from build123d import *

# Parameters (mm, degrees)
SKETCH_1_R          = 12.5
SKETCH_1_R_2        = 3.05
EXTRUDE_1_DEPTH     = 8
SKETCH_2_R          = 1.6
CUT_EXTRUDE_4_DEPTH = 12.5
SKETCH_3_R          = 5.05
EXTRUDE_2_DEPTH     = 6
SKETCH_4_R          = 18
EXTRUDE_3_DEPTH     = 2
FILLET_2_R          = 30
FILLET_1_R          = 1
EXTRUDE_4_DEPTH     = 10
FILLET_3_R          = 4
SKETCH_6_R          = 3.05
CUT_EXTRUDE_5_DEPTH = 14
CUT_EXTRUDE_6_REACH = 81.906


with BuildPart() as part:
    # 草图1 → 凸台-拉伸1 (new body)
    with BuildSketch(Plane(origin=(0, 0, 0), x_dir=(1, 0, 0), z_dir=(0, 1, 0))):
        with Locations(Location((0, 0, 0), (0, 0, 270))):
            Circle(SKETCH_1_R)
        with Locations(Location((0, 0, 0), (0, 0, 270))):
            Circle(SKETCH_1_R_2, mode=Mode.SUBTRACT)
    extrude(amount=EXTRUDE_1_DEPTH)

    # 草图2 → 切除-拉伸4 (cut, symmetric)
    with BuildSketch(Plane.XY):
        with Locations((0, 3.3)):
            Circle(SKETCH_2_R)
    extrude(amount=CUT_EXTRUDE_4_DEPTH, both=True, mode=Mode.SUBTRACT)

    # 草图3 → 凸台-拉伸2 (add)
    with BuildSketch(Plane(origin=(0, 8, 0), x_dir=(1, 0, 0), z_dir=(0, 1, 0))):
        with BuildLine():
            Line((5.416666667, 24.406141076), (62.6, 11.714947716))
            ThreePointArc((62.6, 11.714947716), (71.918087828, 1.399708015), (65.243514508, -10.793773928))
            Line((65.243514508, -10.793773928), (36, -25))
            Line((36, -25), (0, -25))
            ThreePointArc((0, -25), (-24.851091796, 2.724561717), (5.416666667, 24.406141076))
        make_face()
        with Locations(Location((60, 0, 0), (0, 0, 270))):
            Circle(SKETCH_3_R, mode=Mode.SUBTRACT)
    extrude(amount=EXTRUDE_2_DEPTH)

    # 草图4 → 凸台-拉伸3 (add)
    with BuildSketch(Plane.XZ.offset(-8)):
        with Locations(Location((0, 0, 0), (0, 0, 90))):
            Circle(SKETCH_4_R)
    extrude(amount=EXTRUDE_3_DEPTH)

    # 圆角2
    fillet_2_edges = [part.edges().sort_by_distance(p)[0] for p in [
        (36, 11, 25),
    ]]
    fillet(fillet_2_edges, radius=FILLET_2_R)

    # 圆角1
    fillet_1_edges = [part.edges().sort_by_distance(p)[0] for p in [
        (0, 6, -18),
    ]]
    fillet(fillet_1_edges, radius=FILLET_1_R)

    # 草图5 → 凸台-拉伸4 (add)
    with BuildSketch(Plane(origin=(0, 14, 0), x_dir=(1, 0, 0), z_dir=(0, 1, 0))):
        with BuildLine():
            Line((0, 0), (-25, 0))
            ThreePointArc((-25, 0), (-23.096988313, -9.567085809), (-17.67766953, -17.67766953))
            Line((-17.67766953, -17.67766953), (0, 0))
        make_face()
    extrude(amount=EXTRUDE_4_DEPTH)

    # 圆角3
    fillet_3_edges = [part.edges().sort_by_distance(p)[0] for p in [
        (0, 19, 0),
    ]]
    fillet(fillet_3_edges, radius=FILLET_3_R)

    # 草图6 → 切除-拉伸5 (cut)
    with BuildSketch(Plane.XZ):
        with Locations(Location((0, 0, 0), (0, 0, 90))):
            Circle(SKETCH_6_R)
    extrude(amount=-CUT_EXTRUDE_5_DEPTH, mode=Mode.SUBTRACT)

    # 切除-拉伸6: up to this face of the body (flat: up to its plane)
    cut_extrude_6_end = Plane(part.part.faces().sort_by_distance((0, 6, -16.519167389))[0])
    # 草图8 → 切除-拉伸6 (cut, up to the picked face)
    with BuildSketch(Plane.XZ, mode=Mode.PRIVATE) as cut_extrude_6_sk1:
        with BuildLine():
            ThreePointArc((5.937171044, 11), (0, 12.5), (-5.937171044, 11))
            Line((-5.937171044, 11), (5.937171044, 11))
        make_face()
    cut_extrude_6_tool1 = split(extrude(cut_extrude_6_sk1.sketch, amount=-CUT_EXTRUDE_6_REACH, mode=Mode.PRIVATE), bisect_by=cut_extrude_6_end, keep=Keep.BOTH, mode=Mode.PRIVATE)
    # 草图8 → 切除-拉伸6 (cut, up to the picked face)
    with BuildSketch(Plane.XZ, mode=Mode.PRIVATE) as cut_extrude_6_sk2:
        with BuildLine():
            Line((5.937171044, -11), (-5.937171044, -11))
            ThreePointArc((-5.937171044, -11), (0, -12.5), (5.937171044, -11))
        make_face()
    cut_extrude_6_tool2 = split(extrude(cut_extrude_6_sk2.sketch, amount=-CUT_EXTRUDE_6_REACH, mode=Mode.PRIVATE), bisect_by=cut_extrude_6_end, keep=Keep.BOTH, mode=Mode.PRIVATE)
    add(cut_extrude_6_tool1.solids().sort_by(Axis((0, 0, 11.603197), (0, 1, 0)))[0], mode=Mode.SUBTRACT)
    add(cut_extrude_6_tool2.solids().sort_by(Axis((0, 0, -11.603197), (0, 1, 0)))[0], mode=Mode.SUBTRACT)


solid = part.part
The listing builds one solid part. Answer for the finished solid, in the listing's coordinates (mm). A direction names the side the tool comes from. Give positions to 0.01 mm unless a question says otherwise; leave off trailing zeros. Loops run counter-clockwise (first coordinate to the right, second up) from the corner with the lowest first, then second, coordinate; pieces in that order, holes last. Notation, with made-up numbers: (67, 46.5) - (121, 46.5) arc R16 ccw to (121, 50.5) - close; hole circle Ø11 at (16.25, -2.75). An arc over 180 degrees is marked (long way). Answer as a JSON object with one key per item and string values.
1. For faces 1 (the cylindrical face through (12.5, 3, 0.2)), 2 (the flat face through (1.4, 1.6, -11)), 3 (the cylindrical face through (-5.987, 19.07, 2.409)), determine the directions among +Z, -Z, +X, -X, +Y, -Y from which every point of the face is accessible in a straight line to the end or side of a thin tool.
Determined:
{"face 1": "+X, -Y", "face 2": "-Z, +X, -X, -Y", "face 3": "+X, +Y"}
2. Flat-ended cylindrical pins translate along their axes: pin 1 Ø5 at (x, y) = (0, 3.3) entering from -Z; pin 2 Ø3 at (x, y) = (2, 2.5) entering from +Z; pin 3 Ø12 at (x, y) = (21.5, 17) entering from -Z; pin 4 Ø6 at (x, y) = (39.5, 4) entering from +Z. Find the tip coordinate at first contact, or state that the pin passes through.
Determined:
{"pin 1": "z = -11", "pin 2": "z = 11", "pin 3": "z = -21.99", "pin 4": "through"}
3. A cutting plane is placed at C-C (y = 15.5). Write down the section's boundary in (x, z).
Determined:
{"outline": "(-25, 0) - (-9.66, 0) arc R4 ccw to (-6.83, 6.83) - (-17.68, 17.68) arc R25 ccw to start"}
4. Find the intervals of material crossed by L1, parallel to X at y = 9.3, z = 0; L2, parallel to Y at x = 0, z = -7; L3, parallel to Y at x = -7.5, z = -20, in increasing order. Write a range as [from, to].
Determined:
{"L1": "[-25, -3.05], [3.05, 54.95], [65.05, 72]", "L2": "[0, 1.7], [4.9, 14]", "L3": "[8, 14]"}
5. For a pull along X with two mould halves and no side action, classify faces 4 (the flat face through (33.61, 10.96, -18.15)), 5 (the flat face through (-1.4, 1.6, 11)), 6 (the cylindrical face through (55.07, 10.96, -1.09)) as pulls with the +X half, pulls with the -X half, needs draft (parallel to the pull), parting line crosses it, or undercut.
Determined:
{"face 4": "pulls with the +X half", "face 5": "needs draft", "face 6": "undercut"}
6. A cutting plane is placed at A-A (y = 3.3). Write down the section's boundary in (x, z).
Determined:
{"outline": "(-5.94, -11) - (-1.6, -11) - (-1.6, -2.6) arc R3.05 cw to (-1.6, 2.6) - (-1.6, 11) - (-5.94, 11) arc R12.5 ccw to start; (1.6, -11) - (5.94, -11) arc R12.5 ccw to (5.94, 11) - (1.6, 11) - (1.6, 2.6) arc R3.05 cw to (1.6, -2.6) - close"}
7. A cutting plane is placed at B-B (x = 60). Write down the section's boundary in (y, z), then the cut area to 3 significant figures.
Determined:
{"outline": "(8, -12.29) - (14, -12.29) - (14, -5.05) - (8, -5.05) - close; (8, 5.05) - (14, 5.05) - (14, 13.34) - (8, 13.34) - close", "area": "93.2 mm²"}
